from build123d import *

# Parameters (mm, degrees)
SKETCH1_R           = 8.5
SKETCH1_R_2         = 5
BOSS_EXTRUDE1_DEPTH = 10
CUT_EXTRUDE1_DEPTH  = 25
BOSS_EXTRUDE2_DEPTH = 50
CUT_EXTRUDE2_REACH  = 159.194
SKETCH4_R           = 5
CUT_EXTRUDE3_REACH  = 156.975
SKETCH5_W           = 19
SKETCH5_H           = 15
CUT_EXTRUDE4_START  = -17
CUT_EXTRUDE4_DEPTH  = 17
SKETCH7_R           = 4
CUT_EXTRUDE5_DEPTH  = 17
BOSS_EXTRUDE3_REACH = 159.194
SKETCH8_R           = 5


with BuildPart() as part:
    # Sketch1 → Boss-Extrude1 (new, symmetric)
    with BuildSketch(Plane.XY):
        with BuildLine():
            ThreePointArc((10, 130), (0.702455902, 139.975297274), (-9.901311141, 131.401441289))
            Line((-9.901311141, 131.401441289), (-27.380498519, 7.90938056))
            Line((-27.380498519, 7.90938056), (-28.5, 0))
            ThreePointArc((-28.5, 0), (0, -28.5), (28.5, 0))
            Line((28.5, 0), (27.368578637, 7.950528498))
            Line((27.368578637, 7.950528498), (10, 130))
        make_face()
        Circle(SKETCH1_R, mode=Mode.SUBTRACT)
        with Locations((0, 130)):
            Circle(SKETCH1_R_2, mode=Mode.SUBTRACT)
    extrude(amount=BOSS_EXTRUDE1_DEPTH, both=True)

    # Sketch2 → Cut-Extrude1 (cut, symmetric)
    with BuildSketch(Plane(origin=(0, 0, 0), x_dir=(0, 0, -1), z_dir=(1, 0, 0))):
        Polygon((-5, 140), (-10, -28.5), (-10, 140), align=None)
    cut_extrude1 = extrude(amount=CUT_EXTRUDE1_DEPTH, both=True, mode=Mode.SUBTRACT)

    # Mirror1: Cut-Extrude1 across plane
    add(cut_extrude1.mirror(Plane.XY), mode=Mode.SUBTRACT)

    # Sketch3 → Boss-Extrude2 (add)
    with BuildSketch(Plane(origin=(0, 0.271402053, 9.146249197), x_dir=(1, 0, 0), z_dir=(0, 0.02966053500132691, 0.9995600295447169))):
        with BuildLine():
            ThreePointArc((-25, -13.961476874), (0, 28.634294762), (25, -13.961476874))
            add(Edge.make_bspline(
                [(-25, -13.961476874), (0, -59.655586885), (25, -13.961476874)],
                knots=[2.07160832, 2.07160832, 2.07160832, 4.211576987, 4.211576987, 4.211576987], degree=2, weights=[1, 0.480137971, 1]))
        make_face()
    extrude(amount=BOSS_EXTRUDE2_DEPTH)

    # Sketch4 → Cut-Extrude2 (cut, up to next)
    with BuildSketch(Plane(origin=(0, 1.754428803, 59.124250674), x_dir=(1, 0, 0), z_dir=(0, 0.029660535001326913, 0.9995600295447169)), mode=Mode.PRIVATE) as cut_extrude2_sk1:
        with Locations(Location((0, 0, 0), (0, 0, 270))):
            Circle(SKETCH4_R)
    cut_extrude2_tool1 = extrude(cut_extrude2_sk1.sketch, amount=-CUT_EXTRUDE2_REACH, mode=Mode.PRIVATE) & part.part
    add(cut_extrude2_tool1.solids().sort_by_distance((0, 1.754429, 59.124251))[0], mode=Mode.SUBTRACT)

    # Sketch5 → Cut-Extrude3 (cut, up to next)
    with BuildSketch(Plane(origin=(0, 0, 0), x_dir=(1, 0, 0), z_dir=(0, 1, 0)), mode=Mode.PRIVATE) as cut_extrude3_sk1:
        with Locations((0, -17.5)):
            Rectangle(SKETCH5_W, SKETCH5_H)
    cut_extrude3_tool1 = extrude(cut_extrude3_sk1.sketch, amount=-CUT_EXTRUDE3_REACH, mode=Mode.PRIVATE) & part.part
    add(cut_extrude3_tool1.solids().sort_by_distance((0, 0, 17.5))[0], mode=Mode.SUBTRACT)

    # Sketch6 → Cut-Extrude4 (cut)
    with BuildSketch(Plane(origin=(0, 1.754428803, 59.124250674), x_dir=(1, 0, 0), z_dir=(0, 0.029660535001326913, 0.9995600295447168)).offset(CUT_EXTRUDE4_START)):
        with BuildLine():
            ThreePointArc((25, -13.961476874), (0, 28.634294762), (-25, -13.961476874))
            add(Edge.make_bspline(
                [(-25, -13.961476874), (0, -59.655586885), (25, -13.961476874)],
                knots=[2.07160832, 2.07160832, 2.07160832, 4.211576987, 4.211576987, 4.211576987], degree=2, weights=[1, 0.480137971, 1]))
        make_face()
        with BuildLine():
            add(Edge.make_bspline(
                [(-11.871872779, -6.70467228), (-11.297921787, -7.765822714), (-9.855955264, -9.743319402), (-6.038165372, -12.782735574), (0, -14.451619937), (6.038165372, -12.782735574), (9.855955264, -9.743319402), (11.297921787, -7.765822714), (11.871872779, -6.70467228)],
                knots=[2.06679188, 2.06679188, 2.06679188, 2.06679188, 2.335492074, 2.604192267, 3.141592654, 3.67899304, 3.947693234, 4.216393427, 4.216393427, 4.216393427, 4.216393427], degree=3))
            ThreePointArc((11.871872779, -6.70467228), (0, 13.634294762), (-11.871872779, -6.70467228))
        make_face(mode=Mode.SUBTRACT)
    extrude(amount=CUT_EXTRUDE4_DEPTH, mode=Mode.SUBTRACT)

    # Sketch7 → Cut-Extrude5 (cut)
    with BuildSketch(Plane(origin=(0, 1.250199708, 42.131730172), x_dir=(1, 0, 0), z_dir=(0, 0.029660535001326933, 0.9995600295447168))):
        with Locations(Location((20.634294762, 0, 0), (0, 0, 270))):
            Circle(SKETCH7_R)
        with Locations(Location((0.15140188, -20.783506756, 0), (0, 0, 270))):
            Circle(SKETCH7_R)
        with Locations(Location((-20.632104876, -0.300613874, 0), (0, 0, 270))):
            Circle(SKETCH7_R)
        with Locations(Location((-0.149211994, 20.482892882, 0), (0, 0, 270))):
            Circle(SKETCH7_R)
    extrude(amount=-CUT_EXTRUDE5_DEPTH, mode=Mode.SUBTRACT)

    # Boss-Extrude3: up to this face of the body (flat: up to its plane)
    boss_extrude3_end = Plane(part.part.faces().sort_by_distance((-1e-09, -14.541060852, 25))[0])
    # Sketch8 → Boss-Extrude3 (add, up to the picked face)
    with BuildSketch(Plane(origin=(0, 1.754428803, 59.124250674), x_dir=(1, 0, 0), z_dir=(0, 0.029660535001326913, 0.9995600295447168)), mode=Mode.PRIVATE) as boss_extrude3_sk1:
        with Locations(Location((0, 0, 0), (0, 0, 270))):
            Circle(SKETCH8_R)
    boss_extrude3_tool1 = split(extrude(boss_extrude3_sk1.sketch, amount=-BOSS_EXTRUDE3_REACH, mode=Mode.PRIVATE), bisect_by=boss_extrude3_end, keep=Keep.BOTH, mode=Mode.PRIVATE)
    add(boss_extrude3_tool1.solids().sort_by(Axis((0, 1.754429, 59.124251), (0, -0.029660535001326913, -0.9995600295447168)))[0])


solid = part.part
Source: CAD feature listing. Evaluate the final solid. Frame: model axes, mm. A direction names the side the tool comes from. Round coordinates to 2 decimals unless told otherwise and drop trailing zeros. Loops run counter-clockwise (first coordinate to the right, second up) from the corner with the lowest first, then second, coordinate; pieces in that order, holes last. Notation, with made-up numbers: (38, 45.25) - (82, 45.25) arc R17 ccw to (82, 69.25) - close; hole circle Ø5 at (-20, -15). An arc over 180 degrees is marked (long way). Write item = value, one per line. Start each with the question number.
(1) Set-up query: faces 4 (the face through (-0.627, -28.493, 0.14)), 5 (the face through (-0.651, 134.957, -0.077)), 6 (the face through (0, -15, 25)). Return all of +Z, -Z, +X, -X, +Y, -Y with unobstructed straight access to the full face (end or side cutting, diameter ignored); none if empty.
(2) Section query A-A, the plane y = 33.5. Output: boundary loops of the cut face in (x, z).
(3) Pull-direction query (Y, two-part tool) for faces 1 (the face through (-1.68, 17.78, 33.26)), 2 (the face through (-0.834, 29.364, 24.559)), 3 (the face through (-26, 2, -10)); classes: +Y half, -Y half, draft (parallel to the pull), parting line (faces both ways), or undercut.
(4) Pin query (flat end, axial travel): pin 1 (1.1 mm diameter, centred on x = 26.5, y = 15, fed in from +Z); pin 2 (6 mm diameter, centred on y = 75.5, z = 8, fed in from -X); pin 3 (6 mm diameter, centred on x = 20.5, z = 2, fed in from -Y). Return the tip coordinate at first contact, or that it passes through.
(5) Section query B-B, the plane z = 29. State how many separate pieces and enclosed holes the cut face has, plus the area to 3 significant figures.
(6) Section query C-C, the plane y = 59. Output: boundary loops of the cut face in (x, z).
(7) Ray query, line 1 along X through (y, z) = (0, 3.25); line 2 along Y through (x, z) = (0.5, 34); line 3 along X through (y, z) = (130, 0.25). Return the intervals inside material, ascending. Write a range as from..to.
Conclusion:
q1.face_4 = -Z, -Y
q1.face_5 = +Z, -Z
q1.face_6 = -Y
q2.outline = (-23.76, -8.16) - (23.73, -8.16) - (23.73, 8.16) - (-23.76, 8.16) - close
q3.face_1 = undercut
q3.face_2 = parting line
q3.face_3 = draft
q4.pin_1 = 10
q4.pin_2 = -18.21
q4.pin_3 = -22.49
q5.separate_pieces = 1
q5.enclosed_holes = 4
q5.area = 2,380 mm2
q6.outline = (-20.15, -7.4) - (20.1, -7.4) - (20.1, 7.4) - (-20.15, 7.4) - close
q7.line_1 = -28.5..-8.5, 8.5..28.5
q7.line_2 = -27.78..-23.77, -15.8..17.55, 25.45..29.65
q7.line_3 = -10.1..-5, 5..10
